from build123d import *

# Parameters (mm, degrees)
SKETCH2_W           = 12
SKETCH2_H           = 19
BOSS_EXTRUDE1_DEPTH = 3.1115


with BuildPart() as part:
    # Sketch2 → Boss-Extrude1 (new body)
    with BuildSketch(Plane.XY):
        with BuildLine():
            Line((-5.168924328, -39.869822198), (-5.168924328, -33.369822198))
            Line((-5.168924328, -33.369822198), (-12.168924328, -33.369822198))
            add(Edge.make_bspline(
                [(-12.168924328, -33.369822198), (-13.552096669, -33.459867166), (-16.039644903, -35.695120164), (-16.470924328, -39.869822198)],
                knots=[0, 0, 0, 0, 1, 1, 1, 1], degree=3))
            Line((-16.470924328, -39.869822198), (-23.168924328, -39.869822198))
            Line((-23.168924328, -39.869822198), (-23.168924328, -33.469822198))
            Line((-23.168924328, -33.469822198), (-23.168924328, -29.869822198))
            Line((-23.168924328, -29.869822198), (-20.970924328, -29.869822198))
            Line((-20.970924328, -29.869822198), (-20.970924328, -32.069822198))
            Line((-20.970924328, -32.069822198), (-17.970924328, -32.069822198))
            Line((-17.970924328, -32.069822198), (-17.970924328, -29.869822198))
            Line((-17.970924328, -29.869822198), (-16.470924328, -29.869822198))
            Line((-16.470924328, -29.869822198), (-16.470924328, -26.269822198))
            Line((-16.470924328, -26.269822198), (-17.970924328, -26.269822198))
            Line((-17.970924328, -26.269822198), (-17.970924328, -24.069822198))
            Line((-17.970924328, -24.069822198), (-20.970924328, -24.069822198))
            Line((-20.970924328, -24.069822198), (-20.970924328, -26.269822198))
            Line((-20.970924328, -26.269822198), (-23.168924328, -26.269822198))
            Line((-23.168924328, -26.269822198), (-23.168924328, -20.869822198))
            Line((-23.168924328, -20.869822198), (-26.470924328, -20.869822198))
            Line((-26.470924328, -20.869822198), (-26.470924328, -8.869822198))
            Line((-26.470924328, -8.869822198), (-23.168924328, -8.869822198))
            Line((-23.168924328, -8.869822198), (-23.168924328, 0.130177802))
            Line((-23.168924328, 0.130177802), (-20.979823214, 0.130177802))
            Line((-20.979823214, 0.130177802), (-20.970924328, 0.130177802))
            Line((-20.970924328, 0.130177802), (-20.970924328, -2.069822198))
            Line((-20.970924328, -2.069822198), (-17.970924328, -2.069822198))
            Line((-17.970924328, -2.069822198), (-17.970924328, 0.130177802))
            Line((-17.970924328, 0.130177802), (-16.470924328, 0.130177802))
            Line((-16.470924328, 0.130177802), (-16.470924328, 3.730177802))
            Line((-16.470924328, 3.730177802), (-17.970924328, 3.730177802))
            Line((-17.970924328, 3.730177802), (-17.970924328, 5.930177802))
            Line((-17.970924328, 5.930177802), (-20.970924328, 5.930177802))
            Line((-20.970924328, 5.930177802), (-20.970924328, 3.730177802))
            Line((-20.970924328, 3.730177802), (-20.979823214, 3.730177802))
            Line((-20.979823214, 3.730177802), (-23.168924328, 3.730177802))
            Line((-23.168924328, 3.730177802), (-23.168924328, 10.130177802))
            Line((-23.168924328, 10.130177802), (-23.168924328, 17.130177802))
            Line((-23.168924328, 17.130177802), (48.831075672, 17.130177802))
            Line((48.831075672, 17.130177802), (48.831075672, 10.130177802))
            Line((48.831075672, 10.130177802), (48.831075672, 3.730177802))
            Line((48.831075672, 3.730177802), (46.641974559, 3.730177802))
            Line((46.641974559, 3.730177802), (46.633075672, 3.730177802))
            Line((46.633075672, 3.730177802), (46.633075672, 5.930177802))
            Line((46.633075672, 5.930177802), (43.633075672, 5.930177802))
            Line((43.633075672, 5.930177802), (43.633075672, 3.730177802))
            Line((43.633075672, 3.730177802), (42.133075672, 3.730177802))
            Line((42.133075672, 3.730177802), (42.133075672, 0.130177802))
            Line((42.133075672, 0.130177802), (43.633075672, 0.130177802))
            Line((43.633075672, 0.130177802), (43.633075672, -2.069822198))
            Line((43.633075672, -2.069822198), (46.633075672, -2.069822198))
            Line((46.633075672, -2.069822198), (46.633075672, 0.130177802))
            Line((46.633075672, 0.130177802), (46.641974559, 0.130177802))
            Line((46.641974559, 0.130177802), (48.831075672, 0.130177802))
            Line((48.831075672, 0.130177802), (48.831075672, -3.469822198))
            Line((48.831075672, -3.469822198), (48.831075672, -6.869822198))
            Line((48.831075672, -6.869822198), (48.831075672, -8.869822198))
            Line((48.831075672, -8.869822198), (52.133075672, -8.869822198))
            Line((52.133075672, -8.869822198), (52.133075672, -20.869822198))
            Line((52.133075672, -20.869822198), (48.831075672, -20.869822198))
            Line((48.831075672, -20.869822198), (48.831075672, -22.869822198))
            Line((48.831075672, -22.869822198), (48.831075672, -26.269822198))
            Line((48.831075672, -26.269822198), (46.633075672, -26.269822198))
            Line((46.633075672, -26.269822198), (46.633075672, -24.069822198))
            Line((46.633075672, -24.069822198), (43.633075672, -24.069822198))
            Line((43.633075672, -24.069822198), (43.633075672, -26.269822198))
            Line((43.633075672, -26.269822198), (42.133075672, -26.269822198))
            Line((42.133075672, -26.269822198), (42.133075672, -29.869822198))
            Line((42.133075672, -29.869822198), (43.633075672, -29.869822198))
            Line((43.633075672, -29.869822198), (43.633075672, -32.069822198))
            Line((43.633075672, -32.069822198), (46.633075672, -32.069822198))
            Line((46.633075672, -32.069822198), (46.633075672, -29.869822198))
            Line((46.633075672, -29.869822198), (48.831075672, -29.869822198))
            Line((48.831075672, -29.869822198), (48.831075672, -39.869822198))
            Line((48.831075672, -39.869822198), (42.133075672, -39.869822198))
            add(Edge.make_bspline(
                [(37.831075672, -33.369822198), (39.214248014, -33.459867166), (41.701796248, -35.695120164), (42.133075672, -39.869822198)],
                knots=[0, 0, 0, 0, 1, 1, 1, 1], degree=3))
            Line((37.831075672, -33.369822198), (30.831075672, -33.369822198))
            Line((30.831075672, -33.369822198), (30.831075672, -39.869822198))
            Line((30.831075672, -39.869822198), (-5.168924328, -39.869822198))
        make_face()
        with Locations((12.831075672, 0.630177802)):
            Rectangle(SKETCH2_W, SKETCH2_H, mode=Mode.SUBTRACT)
    extrude(amount=BOSS_EXTRUDE1_DEPTH)


solid = part.part
Here's how the part is built. I have some questions about the finished solid (model axes, mm). A direction names the side the tool comes from. Give positions to 0.01 mm unless a question says otherwise; leave off trailing zeros. Loops run counter-clockwise (first coordinate to the right, second up) from the corner with the lowest first, then second, coordinate; pieces in that order, holes last. Notation, with made-up numbers: (81.5, -30) -> (133.5, -30) arc R14 ccw to (133.5, -7) -> close; hole circle Ø7 at (35, -16.75). An arc over 180 degrees is marked (long way). Answer as a JSON object with one key per item and string values. Group by question number.
Item 1: Will these pins go through, and if not, where does the flat tip stop? pin 1 (1.8 mm diameter, centred on y = -25.5, z = 2, fed in from +X); pin 2 (1 mm diameter, centred on y = -23.5, z = 2.5, fed in from -X); pin 3 (0.9 mm diameter, centred on x = -24, z = 1.5, fed in from -Y).
Item 2: Imagine slicing it at C-C on y = 12. Write out the boundary of the cut face in (x, z).
Item 3: Imagine slicing it at A-A on y = -4. Write out the boundary of the cut face in (x, z), then the cut area to 3 significant figures.
Item 4: Thinking about a two-plate mould opening in Y: for faces 5 (the flat face through (45, -2.07, 2)), 6 (the flat face through (13, -39.87, 2)), 7 (the flat face through (30.831, -37, 2)), 8 (the flat face through (-22, 0.13, 2)), which applies, pulls with the +Y half, pulls with the -Y half, needs draft (parallel to the pull), parting line crosses it, or undercut?
Item 5: Imagine slicing it at B-B on x = 12. Write out the boundary of the cut face in (y, z), then the cut area to 3 significant figures.
Item 6: On a 3-axis mill with a long thin cutter (end or side, diameter ignored), from which of +Z, -Z, +X, -X, +Y, -Y can I reach the whole of each face in a straight line? I mean faces 1 (the flat face through (-23.169, -35, 2)), 2 (the flat face through (-17, -29.87, 2)), 3 (the flat face through (-25, -8.87, 2)), 4 (the flat face through (42.133, 2, 2)). Say none if no direction works.
Item 7: I need wall thicknesses on L1, parallel to Y at x = -20.5, z = 2.1; L2, parallel to X at y = 4, z = 1.4; L3, parallel to Y at x = 8.5, z = 1.4. Which ranges of each line are inside material? Lowest first, please.
Answer list:
{
 "1": {"pin 1": "stops at x = 48.83", "pin 2": "stops at x = -23.17", "pin 3": "stops at y = -20.87"},
 "2": {"outline": "(-23.17, 0) -> (48.83, 0) -> (48.83, 3.11) -> (-23.17, 3.11) -> close"},
 "3": {"outline": "(-23.17, 0) -> (6.83, 0) -> (6.83, 3.11) -> (-23.17, 3.11) -> close; (18.83, 0) -> (48.83, 0) -> (48.83, 3.11) -> (18.83, 3.11) -> close", "area": "187 mm2"},
 "4": {"face 5": "undercut", "face 6": "pulls with the -Y half", "face 7": "needs draft", "face 8": "undercut"},
 "5": {"outline": "(-39.87, 0) -> (-8.87, 0) -> (-8.87, 3.11) -> (-39.87, 3.11) -> close; (10.13, 0) -> (17.13, 0) -> (17.13, 3.11) -> (10.13, 3.11) -> close", "area": "118 mm2"},
 "6": {"face 1": "+Z, -Z, -X, -Y", "face 2": "+Z, -Z, -X", "face 3": "+Z, -Z, -X, +Y", "face 4": "+Z, -Z, +X"},
 "7": {"L1": "y = -39.87 to -32.07, -24.07 to -2.07, 5.93 to 17.13", "L2": "x = -23.17 to -20.97, -17.97 to 6.83, 18.83 to 43.63, 46.63 to 48.83", "L3": "y = -39.87 to -8.87, 10.13 to 17.13"}
}
